Input: part model. Units: mm. Frame: model coordinates. A direction names the side the tool comes from. Round coordinates to 2 decimals unless told otherwise and drop trailing zeros. Loops run counter-clockwise (first coordinate to the right, second up) from the corner with the lowest first, then second, coordinate; pieces in that order, holes last.
(1) Access query for faces 1 (the face through (7.037, 0, 17)), 2 (the face through (12.037, 0, 17)), 3 (the face through (-18.396, 20.975, 0.07)). Directions: +Z, -Z, +X, -X, +Y, -Y. A direction counts if a zero-diameter tool reaches every point of the face in a straight line with its end or side. Return the directions, or none.
(2) Line query: line 1 (X direction, y = -5, z = 17.5); line 2 (Y direction, x = 19, z = 3); line 3 (Y direction, x = -39.5, z = -0.5). Output: solid intervals per line, ascending.
(3) Cut plane D-D, the plane z = -1. Output: boundary loops of the cut face in (x, y), and give its area (3 significant figures).
(4) Draft query along X for faces 4 (the face through (14, 21.583, 4)), 5 (the face through (8.463, 0.302, 28.496)), 6 (the face through (-44.4, -23.9, -0.1)), 7 (the face through (-44.4, 23.9, -0.1)). Return one class per face: released by +X, released by -X, zero draft, split by the parting line, or undercut.
(5) Cut plane A-A, the plane z = 15. Output: boundary loops of the cut face in (x, y), and give its area (3 significant figures).
(6) Cut plane B-B, the plane x = -9.5. Output: boundary loops of the cut face in (y, z).
(7) First-contact query: pin 1 Ø5.5 at (x, y) = (15, 3.5) entering from +Z; pin 2 Ø4 at (y, z) = (6.5, 22.5) entering from -X; pin 3 Ø24.5 at (x, y) = (-29.5, 5.5) entering from +Z; pin 4 Ø17.5 at (x, z) = (5.5, 10) entering from +Y. Flat tips, straight axial feed; report the tip coordinate or a pass-through.
from build123d import *

# Parameters (mm, degrees)
F0_W          = 5
F0_H          = 43.1665030722
F0_W_2        = 11
F1_DEPTH      = 5
F1_DEPTH_BACK = 5
F2_T1_DEPTH   = 51.4213562373
F2_T3_DEPTH   = 27.589671948
F3_W          = 5
F3_H          = 43.1665030722
F4_DEPTH      = 25
F5_R          = 4.99999


# Not quite as in the source:
# - a fillet or chamfer that OpenCascade refuses, or shapes differently, is made with other operations: its cross-section is extruded or revolved along the edge and cut away or added
# - a fillet or chamfer is up to 0.001 mm smaller than in the source, because OpenCascade refuses the exact size
# - a feature names something its author has since deleted; it is built from what else it names


with BuildPart() as f1:
    # F0 (on Top) → F1 (new body, two sides)
    with BuildSketch(Plane.XY) as f1_sk:
        with BuildLine():
            ThreePointArc((-7.0367619663, -1.3552663468), (-21.4300874517, -22.6556162733), (-47, -20))
            Line((-47, -20), (-47, -29.3938769134))
            ThreePointArc((-47, -29.3938769134), (-25.6700714676, -32.3872197753), (-7.0367619663, -21.5832515361))
            Line((-7.0367619663, -21.5832515361), (-7.0367619663, -1.3552663468))
        make_face()
        with BuildLine():
            Line((-7.0367619663, 1.3552663468), (-7.0367619663, -1.3552663468))
            ThreePointArc((-7.0367619663, -1.3552663468), (-7, 0), (-7.0367619663, 1.3552663468))
        make_face()
        with BuildLine():
            ThreePointArc((-7.0367619663, 1.3552663468), (-7, 0), (-7.0367619663, -1.3552663468))
            Line((-7.0367619663, -1.3552663468), (-7.0367619663, -21.5832515361))
            ThreePointArc((-7.0367619663, -21.5832515361), (1, 0), (-7.0367619663, 21.5832515361))
            Line((-7.0367619663, 21.5832515361), (-7.0367619663, 1.3552663468))
        make_face()
        with BuildLine():
            ThreePointArc((-47, 20), (-21.4300874517, 22.6556162733), (-7.0367619663, 1.3552663468))
            Line((-7.0367619663, 1.3552663468), (-7.0367619663, 21.5832515361))
            ThreePointArc((-7.0367619663, 21.5832515361), (-25.6700714676, 32.3872197753), (-47, 29.3938769134))
            Line((-47, 29.3938769134), (-47, 20))
        make_face()
        with BuildLine():
            ThreePointArc((-7.0367619663, 21.5832515361), (1, 0), (-7.0367619663, -21.5832515361))
            Line((-7.0367619663, -21.5832515361), (7.0367619663, -21.5832515361))
            Line((7.0367619663, -21.5832515361), (7.0367619663, 21.5832515361))
            Line((7.0367619663, 21.5832515361), (-7.0367619663, 21.5832515361))
        make_face()
        with Locations((9.5367619663, 0)):
            Rectangle(F0_W, F0_H)
        with Locations((17.5367619663, 0)):
            Rectangle(F0_W_2, F0_H)
        with Locations((25.5367619663, 0)):
            Rectangle(F0_W, F0_H)
    extrude(amount=F1_DEPTH)
    extrude(f1_sk.sketch, amount=-F1_DEPTH_BACK)

    # F2: fillet of radius 5 on 4 edges, made by hand

    # F2_s2 → F2_t1 (cut)
    with BuildSketch(Plane.XY.offset(-25.7106781187)):
        with BuildLine():
            ThreePointArc((-40.3333333333, 23.5702260396), (-44.8867513459, 24.2017883428), (-47, 28.2842712475))
            Line((-47, 28.2842712475), (-47, 20))
            ThreePointArc((-47, 20), (-43.8024463398, 22.0386537791), (-40.3333333333, 23.5702260396))
        make_face()
        with BuildLine():
            ThreePointArc((-40.3333333333, -23.5702260396), (-44.8867513459, -24.2017883428), (-47, -28.2842712475))
            Line((-47, -28.2842712475), (-47, -20))
            ThreePointArc((-47, -20), (-43.8024463398, -22.0386537791), (-40.3333333333, -23.5702260396))
        make_face()
    extrude(amount=F2_T1_DEPTH, mode=Mode.SUBTRACT)

    # F2_s4 → F2_t3 (cut)
    with BuildSketch(Plane.XY.offset(-13.794835974)):
        with BuildLine():
            ThreePointArc((-43.7857142857, -30.8236425293), (-46.1187723552, -28.9881272088), (-47, -26.1533936612))
            Line((-47, -26.1533936612), (-47, -29.3938769134))
            ThreePointArc((-47, -29.3938769134), (-45.4119230492, -30.1516221806), (-43.7857142857, -30.8236425293))
        make_face()
        with BuildLine():
            ThreePointArc((-47, 26.1533936612), (-46.1187723552, 28.9881272088), (-43.7857142857, 30.8236425293))
            ThreePointArc((-43.7857142857, 30.8236425293), (-45.4119230492, 30.1516221806), (-47, 29.3938769134))
            Line((-47, 29.3938769134), (-47, 26.1533936612))
        make_face()
    extrude(amount=F2_T3_DEPTH, mode=Mode.SUBTRACT)

    # F3 (on face) → F4 (join)
    with BuildSketch(Plane.XY.offset(5)):
        with Locations((9.5367619663, 0)):
            Rectangle(F3_W, F3_H)
        with Locations((25.5367619663, 0)):
            Rectangle(F3_W, F3_H)
    extrude(amount=F4_DEPTH)

    # F5 (radius 5 in the source; OpenCascade refuses exactly that, so slightly less here)
    f5_edges = [f1.edges().sort_by_distance(p)[0] for p in [
        (7.036762, 0, 5),
        (7.036762, 0, 30),
        (28.036762, 0, 30),
        (28.036762, 0, -5),
    ]]
    fillet(f5_edges, radius=F5_R)


solid = f1.part
Reported:
1. face 1: +Z, -X, +Y, -Y
1. face 2: +Z, +Y, -Y
1. face 3: +Z, -Z
2. line 1: x = 7.04 to 12.04, 23.04 to 28.04
2. line 2: y = -21.58 to 21.58
2. line 3: y = -32.14 to -23.85, 23.85 to 32.14
3. outline: (-46.89, -27.22) arc R5 ccw to (-43.79, -30.82) arc R33 ccw to (-7.04, -21.58) - (27.94, -21.58) - (27.94, 21.58) - (-7.04, 21.58) arc R33 ccw to (-43.79, 30.82) arc R5 ccw to (-46.89, 27.22) arc R5 ccw to (-40.33, 23.57) arc R25 cw to (-7.04, 1.36) - (-7.04, -1.36) arc R25 cw to (-40.33, -23.57) arc R5 ccw to start
3. area: 2,220 mm2
4. face 4: zero draft
4. face 5: released by -X
4. face 6: undercut
4. face 7: undercut
5. outline: (7.04, -21.58) - (12.04, -21.58) - (12.04, 21.58) - (7.04, 21.58) - close; (23.04, -21.58) - (28.04, -21.58) - (28.04, 21.58) - (23.04, 21.58) - close
5. area: 432 mm2
6. outline: (-24.14, -5) - (-10.9, -5) - (-10.9, 5) - (-24.14, 5) - close; (10.9, -5) - (24.14, -5) - (24.14, 5) - (10.9, 5) - close
7. pin 1: stops at z = 5
7. pin 2: stops at x = 7.04
7. pin 3: passes through
7. pin 4: stops at y = 21.58
